Autodesk Inventor part; units mm, degrees
ref_plane "YZ Plane" through (0, 0, 0) normal (1, 0, 0) x (0, 1, 0)
ref_plane "XZ Plane" through (0, 0, 0) normal (0, 1, 0) x (-1, 0, 0)
ref_plane "XY Plane" through (0, 0, 0) normal (0, 0, 1) x (1, 0, 0)
sketch "Sketch1" plane through (0, 0, 0) normal (0, 0, 1) x (1, 0, 0)
  line L0 (-45, 0) -> (-45, -40) construction
  line L1 (-68, -840) -> (-68, 0) construction
  line L2 (-98, 0) -> (-98, -840) construction
  line L3 (-121, -40) -> (-121, 0) construction
  line L4 (-151, 0) -> (-151, -40) construction
  line L5 (-174, -840) -> (-174, 0) construction
  line L6 (-15, -40) -> (-15, 0) construction
  line L7 (8, 0) -> (8, -840) construction
  line L8 (11, 2) -> (-18, 2)
  line L9 (-18, 2) -> (-18, -18)
  line L10 (-18, -18) -> (-42, -18)
  line L11 (-42, -18) -> (-42, 2)
  line L12 (-42, 2) -> (-71, 2)
  line L13 (-71, 2) -> (-71, -18)
  line L14 (-71, -18) -> (-95, -18)
  line L15 (-95, -18) -> (-95, 2)
  line L16 (-95, 2) -> (-124, 2)
  line L17 (-124, 2) -> (-124, -18)
  line L18 (-124, -18) -> (-148, -18)
  line L19 (-148, -18) -> (-148, 2)
  line L20 (-148, 2) -> (-177, 2)
  line L21 (-177, 2) -> (-177, 42)
  line L22 (-177, 42) -> (11, 42)
  line L23 (11, 42) -> (11, 2)
  point P0 (0, 0)
  dimension "d0" = 60
  dimension "d1" = 40
  dimension "d2" = 2
  dimension "d3" = 3
  dimension "d4" = 3
  dimension "d5" = 3
  dimension "d6" = 3
  dimension "d7" = 3
  dimension "d8" = 3
  dimension "d9" = 3
  dimension "d10" = 3
extrude "Extrusion1" add sketch "Sketch1" against normal blind 40
properties part number "Separator" material "Wood"
Could you check a few things on this model? Use its own coordinates, in mm. A direction names the side the tool comes from. Round coordinates to 2 decimals unless told otherwise and drop trailing zeros. Loops run counter-clockwise (first coordinate to the right, second up) from the corner with the lowest first, then second, coordinate; pieces in that order, holes last. Notation, with made-up numbers: M -6,-21.75 L 47,-21.75 A22 ccw 47,12.25 Z; hole C 30,13.25 d5. An arc over 180 degrees is marked long. Write item = value, one per line.
1. Will these pins go through, and if not, where does the flat tip stop? P1, Ø5, axis at y = -3.5, z = -16, coming from the +X side; P2, Ø6, axis at y = -5, z = -13.5, coming from the -X side; P3, Ø8.5, axis at x = -56, z = -16, coming from the -Y side; P4, Ø22, axis at y = -4, z = -21, coming from the +X side.
Results below:
P1 = -18
P2 = -148
P3 = 2
P4 = 11
2. I want a section at C-C, the plane x = -118.5. Write out the boundary of the cut face in (y, z), and give its area (3 significant figures).
Results below:
outline = M 2,-40 L 42,-40 L 42,0 L 2,0 Z
area = 1,600 mm²
3. I want a section at B-B, the plane z = -3.5. Write out the boundary of the cut face in (x, y).
Results below:
outline = M -177,2 L -148,2 L -148,-18 L -124,-18 L -124,2 L -95,2 L -95,-18 L -71,-18 L -71,2 L -42,2 L -42,-18 L -18,-18 L -18,2 L 11,2 L 11,42 L -177,42 Z
4. Which directions (+Z, -Z, +X, -X, +Y, -Y) give clear straight access to the entire face, cutting with the end or side of a thin tool? Please do faces 4 (the face through (-95, -8, -20)), 5 (the face through (-177, 22, -20)), 6 (the face through (-148, -8, -20)), 7 (the face through (-30, -18, -20)), 8 (the face through (-18, -8, -20)).
Results below:
face_4 = +Z, -Z, -Y
face_5 = +Z, -Z, -X, +Y, -Y
face_6 = +Z, -Z, -X, -Y
face_7 = +Z, -Z, +X, -X, -Y
face_8 = +Z, -Z, +X, -Y
5. I want a section at A-A, the plane y = -2.5. Write out the boundary of the cut face in (x, z), and give its area (3 significant figures).
Results below:
outline = M -148,-40 L -124,-40 L -124,0 L -148,0 Z; M -95,-40 L -71,-40 L -71,0 L -95,0 Z; M -42,-40 L -18,-40 L -18,0 L -42,0 Z
area = 2,880 mm²
6. I need wall thicknesses on probe 1 along X at (y, z) = (-9.5, -11); probe 2 along Y at (x, z) = (2.5, -14). Which ranges of each line are inside material? Lowest first, please.
Results below:
probe_1 = -148 to -124, -95 to -71, -42 to -18
probe_2 = 2 to 42
7. Thinking about a two-plate mould opening in X: for faces 1 (the face through (-42, -8, -20)), 2 (the face through (11, 22, -20)), 3 (the face through (-83, -18, -20)), which applies, +X half, -X half, draft (parallel to the pull), parting line (faces both ways), or undercut?
Results below:
face_1 = undercut
face_2 = +X half
face_3 = draft
